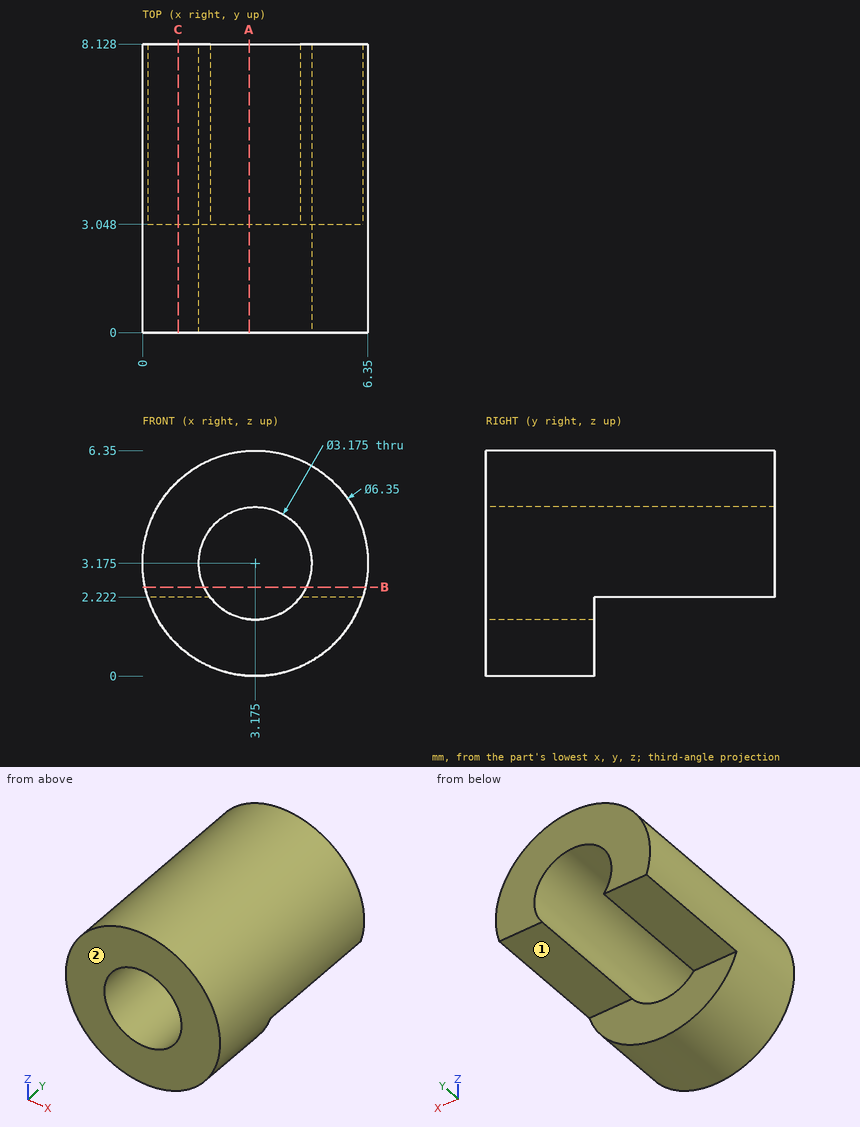
Geometry: see drawing. Coordinates: mm, zero at the bounding-box minimum. A direction names the side the tool comes from. Give positions to 0.01 mm unless a question says otherwise; leave off trailing zeros. Write each loop counter-clockwise with the first axis right and the second up, starting at its lowest first coordinate (ties: lowest second). Pieces come first, ordered by that corner, then holes. Notation, with made-up numbers: M 66,87 L 71,87 A16 ccw 71,91 Z; hole C -16.75,70.25 d4. An arc over 180 degrees is marked long. Return JSON: item names as keys, results as strings. Group by question number.
1) Cut plane C-C, the plane x = 1. Output: boundary loops of the cut face in (y, z), then the cut area to 3 significant figures.
2) Set-up query: the marked faces 1 and 2. Return all of +Z, -Z, +X, -X, +Y, -Y with unobstructed straight access to the full face (end or side cutting, diameter ignored); none if empty.
3) Cut plane A-A, the plane x = 3. Output: boundary loops of the cut face in (y, z) (1 decimal), then the cut area to 3 significant figures.
4) Ray query, L1, parallel to Y at x = 2.25, z = 0.5; L2, parallel to X at y = 3.5, z = 3.75 (1 decimal); L3, parallel to X at y = 0.5, z = 3.5. Return the intervals inside material, ascending.
5) First-contact query: pin 1 Ø1 at (y, z) = (5, 5) entering from -X; pin 2 Ø1.8 at (x, z) = (2.5, 1.5) entering from +Y; pin 3 Ø0.9 at (x, y) = (1.5, 6.5) entering from -Z. Flat tips, straight axial feed; report the tip coordinate or a pass-through.
6) Cut plane B-B, the plane z = 2.5. Output: boundary loops of the cut face in (x, y).
Data:
{
 "1": {"outline": "M 0,0.86 L 3.05,0.86 L 3.05,2.22 L 8.13,2.22 L 8.13,5.49 L 0,5.49 Z", "area": "30.7 mm²"},
 "2": {"face 1": "-Z, +X, -X, +Y", "face 2": "+Z, -Z, +X, -X, -Y"},
 "3": {"outline": "M 0,0 L 3,0 L 3,1.6 L 0,1.6 Z; M 0,4.8 L 8.1,4.8 L 8.1,6.3 L 0,6.3 Z", "area": "17.8 mm²"},
 "4": {"L1": "y = 0 to 3.05", "L2": "x = 0.1 to 1.7, 4.7 to 6.3", "L3": "x = 0.02 to 1.62, 4.73 to 6.33"},
 "5": {"pin 1": "stops at x = 0.29", "pin 2": "stops at y = 3.05", "pin 3": "stops at z = 2.22"},
 "6": {"outline": "M 0.07,0 L 1.74,0 L 1.74,8.13 L 0.07,8.13 Z; M 4.61,0 L 6.28,0 L 6.28,8.13 L 4.61,8.13 Z"}
}
